Design review of the part shown in the three views and the two pictorial views. Dimensions are in mm from the part's minimum x, y and z. A direction names the side the tool comes from. Give positions to 0.01 mm unless a question says otherwise; leave off trailing zeros. Loops run counter-clockwise (first coordinate to the right, second up) from the corner with the lowest first, then second, coordinate; pieces in that order, holes last. Notation, with made-up numbers: (-11.75, 45.25) - (37.25, 45.25) arc R9 cw to (37.25, 61.25) - close; hole circle Ø11 at (3, 72). An arc over 180 degrees is marked (long way). Answer in a Markdown table with one row per item.
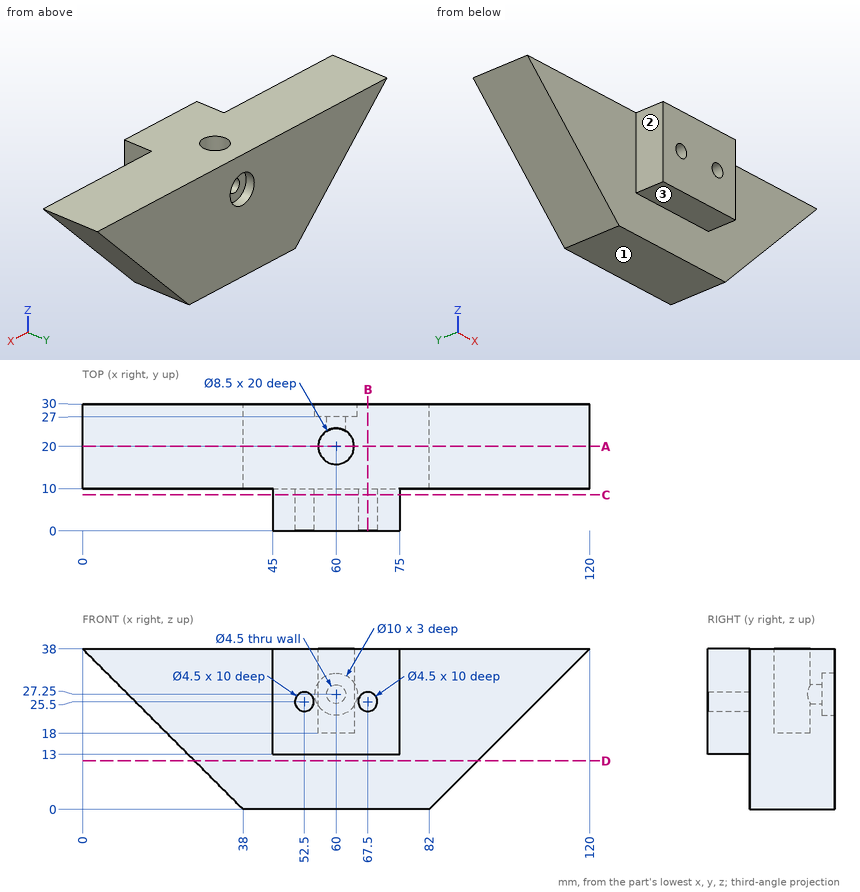
1. Clearance check with flat-ended pins moving along their axes: pin 1 (2.5 mm diameter, centred on x = 62, y = 19.5, fed in from +Z); pin 2 (4 mm diameter, centred on x = 67.5, z = 25.5, fed in from -Y); pin 3 (1.5 mm diameter, centred on y = 20.5, z = 33.5, fed in from -X). State where each tip first meets the part, or that it passes through.
Values:
| item | result |
|---|---|
| pin 1 | stops at z = 18 |
| pin 2 | stops at y = 10 |
| pin 3 | stops at x = 3.75 |
2. Wall thickness on line 1 (X direction, y = 4.75, z = 25.5); line 2 (Z direction, x = 60, y = 25.8); line 3 (Z direction, x = 67.5, y = 3.25): over which ranges is each line inside the solid? List them lowest first. Write a range as [from, to].
Values:
| item | result |
|---|---|
| line 1 | x = [45, 50.25], [54.75, 65.25], [69.75, 75] |
| line 2 | z = [0, 25], [29.5, 38] |
| line 3 | z = [13, 23.25], [27.75, 38] |
3. We need section D-D, the plane z = 11.5. Give the boundary of the cut face in (x, y), and give its area (3 significant figures).
Values:
| item | result |
|---|---|
| outline | (26.5, 10) - (93.5, 10) - (93.5, 30) - (26.5, 30) - close |
| area | 1,340 mm^2 |
4. We need section B-B, the plane x = 67.5. Give the boundary of the cut face in (y, z).
Values:
| item | result |
|---|---|
| outline | (0, 13) - (10, 13) - (10, 0) - (30, 0) - (30, 38) - (0, 38) - (0, 27.75) - (10, 27.75) - (10, 23.25) - (0, 23.25) - close |
5. We need section C-C, the plane y = 8.5. Give the boundary of the cut face in (x, z), and give its area (3 significant figures).
Values:
| item | result |
|---|---|
| outline | (45, 13) - (75, 13) - (75, 38) - (45, 38) - close; hole circle Ø4.5 at (52.5, 25.5); hole circle Ø4.5 at (67.5, 25.5) |
| area | 718 mm^2 |
6. We need section A-A, the plane y = 20. Give the boundary of the cut face in (x, z), and give its area (3 significant figures).
Values:
| item | result |
|---|---|
| outline | (0, 38) - (38, 0) - (82, 0) - (120, 38) - (64.25, 38) - (64.25, 18) - (55.75, 18) - (55.75, 38) - close |
| area | 2,950 mm^2 |
7. For the marked faces 1, 2 and 3, list the 3-axis set-ups (+Z, -Z, +X, -X, +Y, -Y) from which the entire face can be reached by the end or side of a thin tool; tool diameter is ignored.
Values:
| item | result |
|---|---|
| face 1 | -Z, +X, -X, +Y, -Y |
| face 2 | +Z, -Z, -X, -Y |
| face 3 | -Z, +X, -X, -Y |
